Geometry: see drawing. Coordinates: mm, zero at the bounding-box minimum. Coordinates: 2 decimals unless noted, no trailing zeros. Loops run counter-clockwise (first coordinate to the right, second up) from the corner with the lowest first, then second, coordinate; pieces in that order, holes last. Notation, with made-up numbers: (0.5, 57.25) -> (50.5, 57.25) arc R21 ccw to (50.5, 76.25) -> close; hole circle Ø5 at (10.5, 46.5). An arc over 180 degrees is marked (long way). One line per item, written item: value. Start each with the question number.
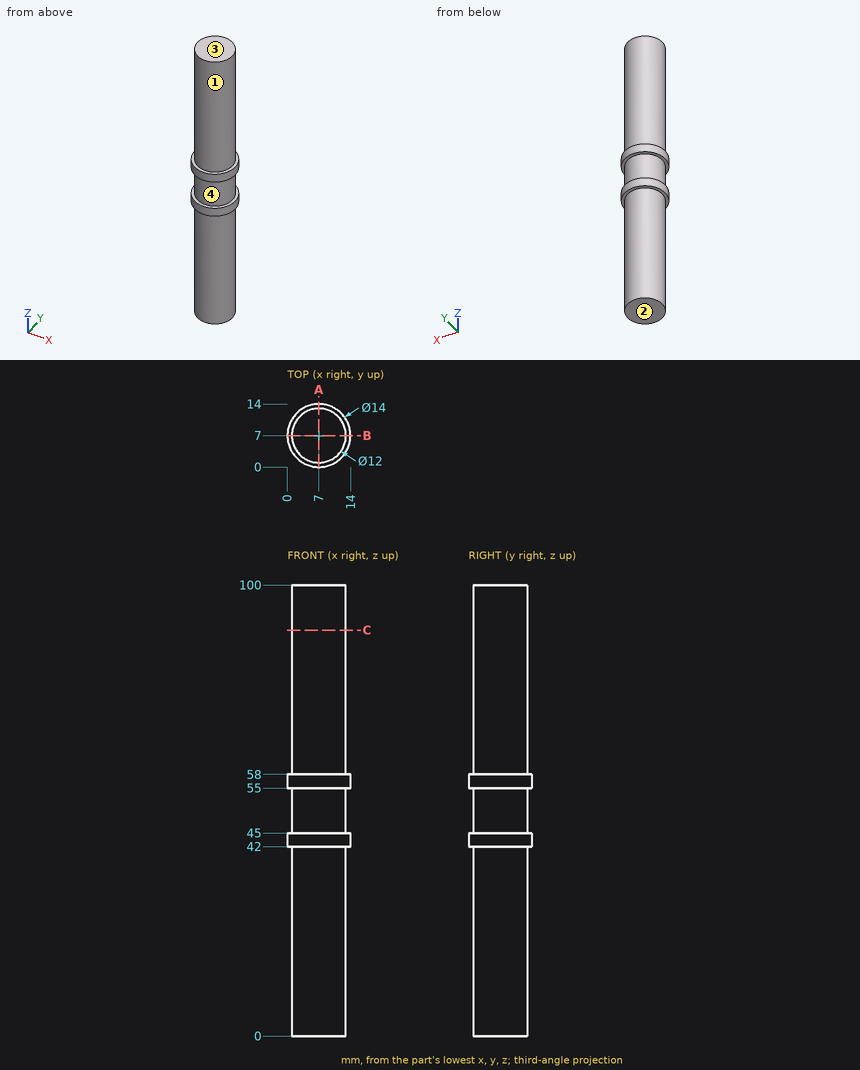
1. Section A-A on x = 7. Return the cut outline in (y, z).
2. Pin query (flat end, axial travel): pin 1 Ø5 at (y, z) = (2.5, 54.5) entering from +X; pin 2 Ø1.5 at (y, z) = (4.5, 36.5) entering from +X; pin 3 Ø5 at (y, z) = (6.5, 51) entering from -X. Return the tip coordinate at first contact, or that it passes through.
3. Line query: L1, parallel to Z at x = 13.25, y = 9; L2, parallel to X at y = 6.75, z = 78.5; L3, parallel to X at y = 3.5, z = 94.5. Output: solid intervals per line, ascending. Write a range as [from, to].
4. Draft query along Z for the marked faces 1, 2, 3 and 4. Return one class per face: released by +Z, released by -Z, zero draft, split by the parting line, or undercut.
5. Section C-C on z = 90. Return the cut outline in (x, y).
Checks:
1. outline: (0, 42) -> (1, 42) -> (1, 0) -> (13, 0) -> (13, 42) -> (14, 42) -> (14, 45) -> (13, 45) -> (13, 55) -> (14, 55) -> (14, 58) -> (13, 58) -> (13, 100) -> (1, 100) -> (1, 58) -> (0, 58) -> (0, 55) -> (1, 55) -> (1, 45) -> (0, 45) -> close
2. pin 1: x = 13.69
2. pin 2: x = 12.74
2. pin 3: x = 1
3. L1: [42, 45], [55, 58]
3. L2: [1.01, 12.99]
3. L3: [2.13, 11.87]
4. face 1: zero draft
4. face 2: released by -Z
4. face 3: released by +Z
4. face 4: undercut
5. outline: circle Ø12 at (7, 7)
